The figure shows three views and two pictorial views of one solid part (mm, origin at its lowest corner). Answer the questions. Give positions to 0.01 mm unless a question says otherwise; leave off trailing zeros. Order: outer loops, then holes, each group sorted by start corner. A loop starts at its lowest first (then second) coordinate and runs counter-clockwise, first axis right, second up. Notation, with made-up numbers: M 73.5,49.5 L 125.5,49.5 A22 cw 125.5,69.5 Z; hole C -5,14 d8. An arc over 180 degrees is marked long. Answer as a JSON object with one key per item and string values. Group by question number.
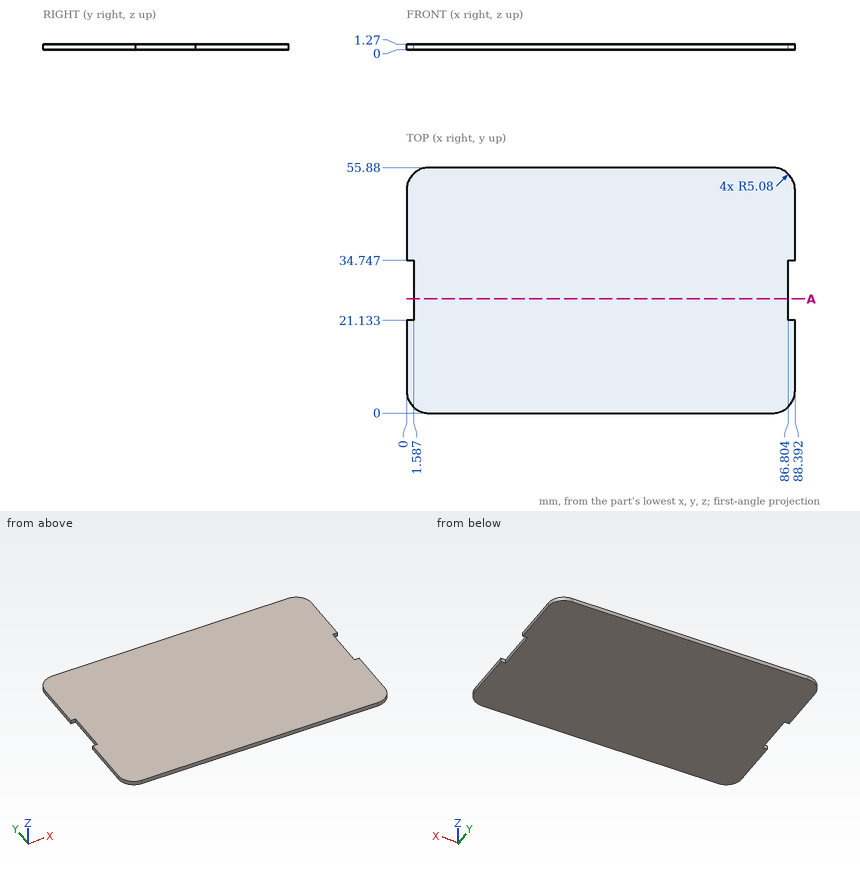
Item 1: Flat-ended cylindrical pins translate along their axes: P1, Ø0.6, axis at x = 87.5, z = 0.5, coming from the -Y side; P2, Ø0.6, axis at y = 27.5, z = 0.5, coming from the +X side (1 decimal); P3, Ø0.6, axis at y = 27.5, z = 1, coming from the -X side. Find the tip coordinate at first contact, or state that the pin passes through.
Item 2: Section A-A (y = 26) is taken. Determine the outline of the cut face in (x, z) (1 decimal), and give its area (3 significant figures).
Item 3: Consider probe 1 along X at (y, z) = (34, 1.2) (1 decimal); probe 2 along Y at (x, z) = (83.5, 0.3). Determine where each line is inside the solid, lowest interval first. Write a range as from..to.
Values found:
{
 "1": {"P1": "stops at y = 1.81", "P2": "stops at x = 86.8", "P3": "stops at x = 1.59"},
 "2": {"outline": "M 1.6,0 L 86.8,0 L 86.8,1.3 L 1.6,1.3 Z", "area": "108 mm^2"},
 "3": {"probe 1": "x = 1.6..86.8", "probe 2": "y = 0..55.88"}
}
